from build123d import *

# Parameters (mm, degrees)
BOSS_EXTRUDE1_DEPTH = 80
SKETCH2_3_W         = 12
SKETCH2_3_H         = 12
BOSS_EXTRUDE2_DEPTH = 3
SKETCH4_R           = 1.5
CUT_EXTRUDE1_DEPTH  = 96.322713731
SKETCH5_R           = 1.5
CUT_EXTRUDE2_DEPTH  = 126.307213604
CUT_EXTRUDE3_DEPTH  = 8
SKETCH7_R           = 1.5
CUT_EXTRUDE5_DEPTH  = 20
BOSS_EXTRUDE3_START = -60
BOSS_EXTRUDE3_DEPTH = 60
CHAMFER1_SIZE       = 5


with BuildPart() as part:
    # Sketch2 → Boss-Extrude1 (new body)
    with BuildSketch(Plane(origin=(0, 0, 0), x_dir=(1, 0, 0), z_dir=(0, 1, 0))):
        Polygon((-80.696905807, 19.555555556), (-95.696905807, 19.555555556), (-95.696905807, 16.555555556), (-83.696905807, 16.555555556), (-83.696905807, 4.555555556), (-35.696905807, 4.555555556), (-35.696905807, 14.555555556), (-80.696905807, 14.555555556), align=None)
    extrude(amount=BOSS_EXTRUDE1_DEPTH)

    # Sketch2<3> → Boss-Extrude2 (add)
    with BuildSketch(Plane(origin=(0, 0, 0), x_dir=(1, 0, 0), z_dir=(0, 1, 0))):
        with Locations((-89.696905807, 10.555555556)):
            Rectangle(SKETCH2_3_W, SKETCH2_3_H)
    extrude(amount=BOSS_EXTRUDE2_DEPTH)

    # Sketch4 → Cut-Extrude1 (cut, through all)
    with BuildSketch(Plane.ZY.offset(83.696905807)):
        with Locations((-9.555555556, 22)):
            Circle(SKETCH4_R)
        with Locations((-9.555555556, 61)):
            Circle(SKETCH4_R)
    extrude(amount=-CUT_EXTRUDE1_DEPTH, mode=Mode.SUBTRACT)

    # Sketch5 → Cut-Extrude2 (cut, through all)
    with BuildSketch(Plane.XY.offset(-16.555555556)):
        with Locations((-90.696905807, 10)):
            Circle(SKETCH5_R)
        with Locations((-90.696905807, 73)):
            Circle(SKETCH5_R)
    extrude(amount=-CUT_EXTRUDE2_DEPTH, mode=Mode.SUBTRACT)

    # Sketch6 → Cut-Extrude3 (cut)
    with BuildSketch(Plane(origin=(0, 0, -14.555555556), x_dir=(-1, 0, 0), z_dir=(0, 0, -1))):
        with BuildLine():
            Line((67.723185249, 52), (70.89861173, 57.5))
            Line((70.89861173, 57.5), (67.723185249, 63))
            ThreePointArc((67.723185249, 63), (58.196905807, 68.5), (48.670626366, 63))
            Line((48.670626366, 63), (45.495199885, 57.5))
            Line((45.495199885, 57.5), (48.670626366, 52))
            ThreePointArc((48.670626366, 52), (58.196905807, 46.5), (67.723185249, 52))
        make_face()
    extrude(amount=-CUT_EXTRUDE3_DEPTH, mode=Mode.SUBTRACT)

    # Sketch7 → Cut-Extrude5 (cut)
    with BuildSketch(Plane(origin=(0, 80, 0), x_dir=(1, 0, 0), z_dir=(0, 1, 0))):
        with Locations(Location((-65.696905807, 9.555555556, 0), (0, 0, 270))):
            Circle(SKETCH7_R)
    extrude(amount=-CUT_EXTRUDE5_DEPTH, mode=Mode.SUBTRACT)

    # Sketch8 → Boss-Extrude3 (add)
    with BuildSketch(Plane(origin=(-35.696905807, 0, 0), x_dir=(0, 0, -1), z_dir=(1, 0, 0)).offset(BOSS_EXTRUDE3_START)):
        with BuildLine():
            Line((14.555555556, 0), (4.501282487, -19.780828807))
            ThreePointArc((4.501282487, -19.780828807), (3.828999817, -20), (3.609828624, -19.32771733))
            Line((3.609828624, -19.32771733), (9.410961448, -7.914538626))
            ThreePointArc((9.410961448, -7.914538626), (9.198154182, -2.598476584), (4.555555556, 0))
            Line((4.555555556, 0), (14.555555556, 0))
        make_face()
    extrude(amount=BOSS_EXTRUDE3_DEPTH)

    # Chamfer1
    chamfer1_edges = [part.edges().sort_by_distance(p)[0] for p in [
        (-80.696905807, 40, -14.555555556),
    ]]
    chamfer(chamfer1_edges, length=CHAMFER1_SIZE - 0.0001)  # a hair under: the kernel refuses the full size


solid = part.part
Geometry check sheet. Reference: the model listing, model coordinates, mm. A direction names the side the tool comes from. Coordinates: 2 decimals unless noted, no trailing zeros. Write each loop counter-clockwise with the first axis right and the second up, starting at its lowest first coordinate (ties: lowest second). Pieces come first, ordered by that corner, then holes. Notation, with made-up numbers: (31, 33) -> (45, 33) arc R31 cw to (45, 67) -> close; hole circle Ø8 at (21, -22.5). An arc over 180 degrees is marked (long way). One line per question, with ' | ' between items.
1. Thickness scan on probe 1 along Y at (x, z) = (-74, -9.25); probe 2 along Z at (x, y) = (-73, 61); probe 3 along Y at (x, z) = (-58, -8.5). Record the ranges inside material, lowest first. Write a range as from..to.
Answers:
probe 1: y = -10.44..-8.23, -2.68..20.53, 23.47..59.53, 62.47..80 | probe 2: z = -14.56..-11.06, -8.06..-4.56 | probe 3: y = -11.91..-9.71, -1.69..20.93, 23.07..46.5, 68.5..80
2. Draft check along Y on faces 1 (the flat face through (-88, 0, -17)), 2 (the cylindrical face through (-60.033, 23.265, -8.749)), 3 (the flat face through (-55, 39, -14.556)). Enter one of: +Y half, -Y half, draft (parallel to the pull), parting line (faces both ways), or undercut.
Answers:
face 1: -Y half | face 2: undercut | face 3: draft
3. Cross-section at C-C on y = 73. State how many separate pieces and enclosed holes the cut face has, and give its area (3 significant figures).
Answers:
separate pieces: 2 | enclosed holes: 1 | area: 527 mm²
4. Depth check by flat-ended pin: pin 1 Ø3.5 at (x, y) = (-88.5, 45.5) entering from +Z; pin 2 Ø12 at (x, y) = (-65.5, 54) entering from -Z; pin 3 Ø2 at (x, z) = (-44.5, -7.5) entering from -Y. Enter the tip coordinate at first touch or a pass-through.
Answers:
pin 1: stops at z = -16.56 | pin 2: stops at z = -14.56 | pin 3: stops at y = -15.85
5. Cross-section at A-A on x = -73.5. Record the cut outline in (y, z), and give its area (3 significant figures).
Answers:
outline: (-19.78, -4.5) -> (0, -14.56) -> (80, -14.56) -> (80, -4.56) -> (0, -4.56) arc R5.45 cw to (-7.91, -9.41) -> (-19.33, -3.61) arc R0.5 ccw to start; hole circle Ø3 at (22, -9.56); hole circle Ø3 at (61, -9.56) | area: 826 mm²
6. Set-up check for faces 4 (the flat face through (-59, 39, -4.556)), 5 (the flat face through (-69.686, 59.6, -10.612)), 6 (the flat face through (-90, 41, -16.556)): record each of +Z, -Z, +X, -X, +Y, -Y from which the full face is reachable in a straight line by a thin tool's end or side.
Answers:
face 4: +Z, +X, -X, +Y | face 5: -Z | face 6: +Z, -X, +Y
